from build123d import *

# Parameters (mm, degrees)
SKETCH1_W           = 430
SKETCH1_H           = 500
BOSS_EXTRUDE1_DEPTH = 1.5
SKETCH12_R          = 1.95
CUT_EXTRUDE3_DEPTH  = 50.8
SKETCH6_R           = 1.95
CUT_EXTRUDE4_DEPTH  = 50.8
SKETCH7_R           = 1.95
CUT_EXTRUDE5_DEPTH  = 50.8
FILLET1_R           = 2
CUT_EXTRUDE6_DEPTH  = 10
SCALE1_SCALE        = 0.76


with BuildPart() as part:
    # Sketch1 → Boss-Extrude1 (new body)
    with BuildSketch(Plane(origin=(0, 0, 0), x_dir=(1, 0, 0), z_dir=(0, 1, 0))):
        Rectangle(SKETCH1_W, SKETCH1_H)
    extrude(amount=BOSS_EXTRUDE1_DEPTH)

    # Sketch12 → Cut-Extrude3 (cut)
    with BuildSketch(Plane(origin=(0, 0, 0), x_dir=(-1, 0, 0), z_dir=(0, -1, 0))):
        with Locations((-185, -175)):
            Circle(SKETCH12_R)
        with Locations((-205, 170)):
            Circle(SKETCH12_R)
        with Locations((-205, -175)):
            Circle(SKETCH12_R)
        with Locations((-185, 170)):
            Circle(SKETCH12_R)
        with Locations((205, -175)):
            Circle(SKETCH12_R)
        with Locations((185, 175)):
            Circle(SKETCH12_R)
        with Locations((205, 175)):
            Circle(SKETCH12_R)
        with Locations((185, -175)):
            Circle(SKETCH12_R)
    extrude(amount=-CUT_EXTRUDE3_DEPTH, mode=Mode.SUBTRACT)

    # Sketch6 → Cut-Extrude4 (cut)
    with BuildSketch(Plane(origin=(0, 1.5, 0), x_dir=(1, 0, 0), z_dir=(0, 1, 0))):
        with Locations((92.292697989, -28)):
            Circle(SKETCH6_R)
        with Locations((42.292697989, -28)):
            Circle(SKETCH6_R)
        with Locations((92.292697989, -178)):
            Circle(SKETCH6_R)
        with Locations((42.292697989, -178)):
            Circle(SKETCH6_R)
    extrude(amount=-CUT_EXTRUDE4_DEPTH, mode=Mode.SUBTRACT)

    # Sketch7 → Cut-Extrude5 (cut)
    with BuildSketch(Plane(origin=(0, 1.5, 0), x_dir=(1, 0, 0), z_dir=(0, 1, 0))):
        with Locations((-114.979961576, 95.192396061)):
            Circle(SKETCH7_R)
        with Locations((-54.979961576, 95.192396061)):
            Circle(SKETCH7_R)
        with Locations((-54.979961576, 0.192396061)):
            Circle(SKETCH7_R)
        with Locations((-114.979961576, 0.192396061)):
            Circle(SKETCH7_R)
    extrude(amount=-CUT_EXTRUDE5_DEPTH, mode=Mode.SUBTRACT)

    # Fillet1
    fillet1_edges = [part.edges().sort_by_distance(p)[0] for p in [
        (215, 0.75, 250),
        (-215, 0.75, 250),
        (-215, 0.75, -250),
        (215, 0.75, -250),
    ]]
    fillet(fillet1_edges, radius=FILLET1_R)

    # Sketch13 → Cut-Extrude6 (cut)
    with BuildSketch(Plane.XZ):
        with BuildLine():
            ThreePointArc((128.328231895, 194.409545443), (128.328231895, 201.480613255), (121.257164083, 201.480613255))
            Line((121.257164083, 201.480613255), (6.257164083, 86.480613255))
            ThreePointArc((6.257164083, 86.480613255), (6.257164083, 79.409545443), (13.328231895, 79.409545443))
            Line((13.328231895, 79.409545443), (128.328231895, 194.409545443))
        make_face()
        with BuildLine():
            ThreePointArc((114.891555161, 206.259007204), (114.891555161, 214.740992796), (106.409569569, 214.740992796))
            Line((106.409569569, 214.740992796), (5.551705193, 113.883128419))
            ThreePointArc((5.551705193, 113.883128419), (5.551705193, 105.401142828), (14.033690785, 105.401142828))
            Line((14.033690785, 105.401142828), (114.891555161, 206.259007204))
        make_face()
        with BuildLine():
            ThreePointArc((128.328231895, 169.409545443), (128.328231895, 176.480613255), (121.257164083, 176.480613255))
            Line((121.257164083, 176.480613255), (6.257164083, 61.480613255))
            ThreePointArc((6.257164083, 61.480613255), (6.257164083, 54.409545443), (13.328231895, 54.409545443))
            Line((13.328231895, 54.409545443), (128.328231895, 169.409545443))
        make_face()
        with BuildLine():
            ThreePointArc((128.328231895, 144.409545443), (128.328231895, 151.480613255), (121.257164083, 151.480613255))
            Line((121.257164083, 151.480613255), (6.257164083, 36.480613255))
            ThreePointArc((6.257164083, 36.480613255), (6.257164083, 29.409545443), (13.328231895, 29.409545443))
            Line((13.328231895, 29.409545443), (128.328231895, 144.409545443))
        make_face()
        with BuildLine():
            ThreePointArc((7.050771569, 137.384062043), (5.156114678, 129.125444121), (13.4147326, 131.020101013))
            Line((13.4147326, 131.020101013), (89.712651072, 207.318019485))
            ThreePointArc((89.712651072, 207.318019485), (89.712651072, 213.681980515), (83.348690041, 213.681980515))
            Line((83.348690041, 213.681980515), (7.050771569, 137.384062043))
        make_face()
        with BuildLine():
            ThreePointArc((128.328231895, 119.409545443), (128.328231895, 126.480613255), (121.257164083, 126.480613255))
            Line((121.257164083, 126.480613255), (6.257164083, 11.480613255))
            ThreePointArc((6.257164083, 11.480613255), (6.257164083, 4.409545443), (13.328231895, 4.409545443))
            Line((13.328231895, 4.409545443), (128.328231895, 119.409545443))
        make_face()
        with BuildLine():
            ThreePointArc((129.178407924, 95.256425689), (129.178407924, 102.327493501), (122.107340112, 102.327493501))
            Line((122.107340112, 102.327493501), (18.815380517, -0.964466094))
            ThreePointArc((18.815380517, -0.964466094), (18.815380517, -8.035533906), (25.886448329, -8.035533906))
            Line((25.886448329, -8.035533906), (129.178407924, 95.256425689))
        make_face()
        with BuildLine():
            ThreePointArc((64.186096271, 206.964466094), (64.186096271, 214.035533906), (57.115028459, 214.035533906))
            Line((57.115028459, 214.035533906), (6.257164083, 163.17766953))
            ThreePointArc((6.257164083, 163.17766953), (6.257164083, 156.106601718), (13.328231895, 156.106601718))
            Line((13.328231895, 156.106601718), (64.186096271, 206.964466094))
        make_face()
        with BuildLine():
            ThreePointArc((128.328231895, 71.106601718), (128.328231895, 78.17766953), (121.257164083, 78.17766953))
            Line((121.257164083, 78.17766953), (42.115028459, -0.964466094))
            ThreePointArc((42.115028459, -0.964466094), (42.115028459, -8.035533906), (49.186096271, -8.035533906))
            Line((49.186096271, -8.035533906), (128.328231895, 71.106601718))
        make_face()
        with BuildLine():
            ThreePointArc((128.434071453, 42.778300689), (128.450410182, 50.077386347), (121.151324524, 50.093725076))
            Line((121.151324524, 50.093725076), (70.101549086, -0.728014801))
            ThreePointArc((70.101549086, -0.728014801), (70.211536159, -8.378376983), (77.854021235, -8.014288369))
            Line((77.854021235, -8.014288369), (80.943634504, -4.5))
            Line((80.943634504, -4.5), (128.434071453, 42.778300689))
        make_face()
        with BuildLine():
            ThreePointArc((39.186096271, 206.964466094), (39.186090231, 214.035539946), (32.11501638, 214.035521827))
            Line((32.11501638, 214.035521827), (28.579518712, 210.5))
            Line((28.579518712, 210.5), (6.257188241, 188.17766953))
            ThreePointArc((6.257188241, 188.17766953), (6.257176162, 181.106613797), (13.328231895, 181.106601718))
            Line((13.328231895, 181.106601718), (39.186096271, 206.964466094))
        make_face()
        with BuildLine():
            ThreePointArc((128.328231895, 21.106601718), (128.328231895, 28.17766953), (121.257164083, 28.17766953))
            Line((121.257164083, 28.17766953), (92.115028459, -0.964466094))
            ThreePointArc((92.115028459, -0.964466094), (92.115028459, -8.035533906), (99.186096271, -8.035533906))
            Line((99.186096271, -8.035533906), (128.328231895, 21.106601718))
        make_face()
        with BuildLine():
            ThreePointArc((128.328449123, -3.893615534), (128.328449135, 3.177669518), (121.257164083, 3.17766953))
            Line((121.257164083, 3.17766953), (117.115028459, -0.964466094))
            ThreePointArc((117.115028459, -0.964466094), (117.11493575, -8.035441194), (124.185910844, -8.035719323))
            Line((124.185910844, -8.035719323), (128.328449123, -3.893615534))
        make_face()
        with BuildLine():
            Line((-60.282225947, -95.192396061), (-54.979961576, -89.89013169))
            Line((-54.979961576, -89.89013169), (-52.328312545, -87.235758493))
            ThreePointArc((-52.328312545, -87.235758493), (-52.33035331, -81.93586188), (-57.630250273, -81.936542135))
            Line((-57.630250273, -81.936542135), (-68.235815502, -92.542107364))
            ThreePointArc((-68.235815502, -92.542107364), (-68.236495757, -97.842004327), (-62.936599144, -97.844045092))
            Line((-62.936599144, -97.844045092), (-60.282225947, -95.192396061))
        make_face()
        with BuildLine():
            Line((-79.432380406, -95.192396061), (-52.328311176, -68.084345475))
            ThreePointArc((-52.328311176, -68.084345475), (-52.332091228, -62.778048343), (-57.638379198, -62.788609103))
            Line((-57.638379198, -62.788609103), (-87.242774375, -92.549084557))
            ThreePointArc((-87.242774375, -92.549084557), (-87.193524879, -97.884311066), (-81.85941362, -97.764626075))
            Line((-81.85941362, -97.764626075), (-79.432380406, -95.192396061))
        make_face()
        with BuildLine():
            Line((-98.589718565, -95.192396061), (-54.979961576, -51.582639071))
            Line((-54.979961576, -51.582639071), (-52.328311176, -48.930599166))
            ThreePointArc((-52.328311176, -48.930599166), (-52.332818712, -43.623576712), (-57.639827781, -43.636319812))
            Line((-57.639827781, -43.636319812), (-106.244222321, -92.550540935))
            ThreePointArc((-106.244222321, -92.550540935), (-106.146641992, -97.928953998), (-100.773557317, -97.670477564))
            Line((-100.773557317, -97.670477564), (-98.589718565, -95.192396061))
        make_face()
        with BuildLine():
            Line((-111.925519092, -89.374450278), (-52.328311147, -29.777242332))
            ThreePointArc((-52.328311147, -29.777242332), (-52.310450744, -24.491922995), (-57.595528665, -24.438342602))
            Line((-57.595528665, -24.438342602), (-117.992839573, -83.224558883))
            ThreePointArc((-117.992839573, -83.224558883), (-118.054977502, -89.353737319), (-111.925519092, -89.374450278))
        make_face()
        with BuildLine():
            Line((-112.328311147, -70.623496023), (-52.374195212, -10.669380088))
            ThreePointArc((-52.374195212, -10.669380088), (-52.374195212, -5.457847361), (-57.58572794, -5.457847361))
            Line((-57.58572794, -5.457847361), (-114.979961576, -62.668544735))
            Line((-114.979961576, -62.668544735), (-117.631612006, -65.320195164))
            ThreePointArc((-117.631612006, -65.320195164), (-117.631612006, -70.623496023), (-112.328311147, -70.623496023))
        make_face()
        with BuildLine():
            Line((-112.328311147, -51.123496023), (-63.949411742, -2.744596618))
            ThreePointArc((-63.949411742, -2.744596618), (-63.936748679, 2.34707829), (-69.028297614, 2.385067165))
            Line((-69.028297614, 2.385067165), (-71.657559216, -0.192396061))
            Line((-71.657559216, -0.192396061), (-114.979961576, -43.514798421))
            Line((-114.979961576, -43.514798421), (-117.432443337, -45.634975273))
            ThreePointArc((-117.432443337, -45.634975273), (-117.726028226, -51.025591461), (-112.328311147, -51.123496023))
        make_face()
        with BuildLine():
            Line((-112.328311147, -31.623496023), (-83.202607923, -2.497792799))
            ThreePointArc((-83.202607923, -2.497792799), (-83.175365618, 2.085432584), (-87.75794332, 2.167155652))
            Line((-87.75794332, 2.167155652), (-117.567824527, -26.25790651))
            ThreePointArc((-117.567824527, -26.25790651), (-117.662945906, -31.591787403), (-112.328311147, -31.623496023))
        make_face()
        with BuildLine():
            Line((-112.328311147, -12.123496023), (-103.048861614, -2.84404649))
            ThreePointArc((-103.048861614, -2.84404649), (-103.048861614, 2.459254369), (-108.352162473, 2.459254369))
            Line((-108.352162473, 2.459254369), (-117.631612006, -6.820195164))
            ThreePointArc((-117.631612006, -6.820195164), (-117.631612006, -12.123496023), (-112.328311147, -12.123496023))
        make_face()
    extrude(amount=-CUT_EXTRUDE6_DEPTH, mode=Mode.SUBTRACT)


with BuildPart() as part_1:
    # Scale1: scaled about (-3.718091903, 0.75, -7.04565373)
    add(part.part.scale(SCALE1_SCALE).moved(Location((-0.892342057, 0.18, -1.690956895))))


solid = part_1.part
Here's how the part is built. I have some questions about the finished solid (model axes, mm). Coordinates: 2 decimals unless noted, no trailing zeros.
1. I need wall thicknesses on L1, parallel to X at y = 0.3, z = -38; L2, parallel to Z at x = -57.5, y = 0.3; L3, parallel to X at y = 0.9, z = 23.5. Which ranges of each line are inside material? Lowest first, please.
2. For P1, Ø2.5, axis at x = -156.69, z = -134.69, coming from the -Y side, with a flat end and sliding along its axis, tell me the tip position at first contact or that it passes through.
3. Imagine slicing it at A-A, the plane y = 0.7. Count the separate pieces of the cut face and the enclosed holes in it, and give its area (3 significant figures).
Taken from the geometry:
1. L1: x = -164.29 to -91.08, -83.72 to -76.92, -68.9 to -62.89, -54.34 to -47.82, -40.06 to 162.51
1. L2: z = -191.69 to -70.28, -62.28 to -55.72, -47.74 to -41.16, -32.76 to -26.6, -18.64 to -11.78, -3.99 to 188.31
1. L3: x = -164.29 to 2.75, 12.08 to 20.33, 31.08 to 39.33, 50.08 to 57.04, 67.79 to 78.24, 89.36 to 162.51
2. P1: passes through
3. separate pieces: 1
3. enclosed holes: 37
3. area: 113,000 mm2
